Here's how the part is built. I have some questions about the finished solid (model axes, mm). A direction names the side the tool comes from. Round coordinates to 2 decimals unless told otherwise and drop trailing zeros. Write each loop counter-clockwise with the first axis right and the second up, starting at its lowest first coordinate (ties: lowest second). Pieces come first, ordered by that corner, then holes. Notation, with made-up numbers: (-36, 47) -> (-25, 47) arc R30 ccw to (-25, 84) -> close; hole circle Ø5 at (82, 58.5). An arc over 180 degrees is marked (long way). Put each result on its own line as item: value. Start each with the question number.
1) I want a section at C-C, the plane x = 59. List the corners of the cut face in (y, z) for me.
2) I want a section at A-A, the plane x = 38.5. List the corners of the cut face in (y, z) for me, then the cut area to 3 significant figures.
3) I want a section at B-B, the plane y = 0.35. Give the number of separate pieces and of enclosed holes in the cut face, then the cut area to 3 significant figures.
4) I want a section at D-D, the plane z = -5. List the corners of the cut face in (x, y) for me, then the cut area to 3 significant figures.
5) Which directions (+Z, -Z, +X, -X, +Y, -Y) give clear straight access to the entire face, cutting with the end or side of a thin tool? Please do faces 1 (the flat face through (5.1, 0.5, 159.9)), 2 (the flat face through (135.876, 0.493, 193.83)).
6) Will this pin go through, and if not, where does the flat tip stop? P1, Ø1.9, axis at x = 114.56, z = 121.63, coming from the -Y side (3 decimals).
7) We'd pull the mould along Z, two halves only. Please class faces 3 (the flat face through (4.93, 0.493, 244.636)), 4 (the flat face through (160, 1, -3)), 5 (the flat face through (5.2, 0.5, -159.8)): released by +Z, released by -Z, zero draft, split by the parting line, or undercut.
8) If I drill on line 1 along Z through (x, y) = (108, 0.6); line 2 along Z through (x, y) = (128, 0.6); line 3 along Z through (x, y) = (105, 0.5), over which ranges is the centre line in solid material (lowest first)? Write a range as [from, to].
from build123d import *

# Parameters (mm, degrees)
EXTRUDE_1_DEPTH     = 1
SKETCH_4_W          = 56.568542495
SKETCH_4_H          = 273.13708499
CUT_EXTRUDE_3_DEPTH = 354.138500868
CHAMFER_1_SIZE      = 10
SKETCH_5_R          = 1.6
CUT_EXTRUDE_4_DEPTH = 10
SKETCH_6_R          = 3
CUT_EXTRUDE_5_DEPTH = 10
SKETCH_7_R          = 1.6
CUT_EXTRUDE_6_DEPTH = 4


with BuildPart() as part:
    # 草图1 → 凸台-拉伸1 (new body)
    with BuildSketch(Plane(origin=(0, 0, 0), x_dir=(1, 0, 0), z_dir=(0, 1, 0))):
        with BuildLine():
            Line((0, 249.705627485), (0, 155))
            ThreePointArc((0, 155), (109.601551084, 109.601551084), (155, 0))
            ThreePointArc((155, 0), (109.601551084, -109.601551084), (0, -155))
            Line((0, -155), (0, -249.705627485))
            Line((0, -249.705627485), (80, -249.705627485))
            Line((80, -249.705627485), (249.705627485, -80))
            Line((249.705627485, -80), (249.705627485, 0))
            Line((249.705627485, 0), (249.705627485, 80))
            Line((249.705627485, 80), (80, 249.705627485))
            Line((80, 249.705627485), (0, 249.705627485))
        make_face()
    extrude(amount=EXTRUDE_1_DEPTH)

    # 草图4 → 切除-拉伸3 (cut, through all)
    with BuildSketch(Plane(origin=(0, 1, 0), x_dir=(1, 0, 0), z_dir=(0, 1, 0))):
        with Locations((221.421356237, 0)):
            Rectangle(SKETCH_4_W, SKETCH_4_H)
    extrude(amount=-CUT_EXTRUDE_3_DEPTH, mode=Mode.SUBTRACT)

    # 倒角1
    # the kernel refuses this chamfer: 10 mm, written as the material it takes off along each edge
    with BuildSketch(Plane(origin=(0, -26.617651024, -155), x_dir=(0.9994423420060535, 0, 0.0333916906648138), z_dir=(0, 1, 0))) as chamfer_1_piece_1:
        with BuildLine():
            Line((10.351424106, 0), (-CHAMFER_1_SIZE * 0.0333916906648, CHAMFER_1_SIZE * 0.999442342006))
            Line((-CHAMFER_1_SIZE * 0.0333916906648, CHAMFER_1_SIZE * 0.999442342006), (0, 0))
            ThreePointArc((0, 0), (5.321987279, 0.086367968), (10.351424106, 0))
        make_face()
    extrude(amount=54.235302047, mode=Mode.SUBTRACT)
    with BuildSketch(Plane(origin=(0, -25.71682988, -249.705627485), x_dir=(0, 0, 1), z_dir=(0, 1, 0))) as chamfer_1_piece_2:
        Polygon((CHAMFER_1_SIZE, 0), (0, CHAMFER_1_SIZE), (0, 0), align=None)
    extrude(amount=52.433659759, mode=Mode.SUBTRACT)
    with BuildSketch(Plane(origin=(80, -25.926703929, -249.705627485), x_dir=(-1, 0, 0), z_dir=(0, 1, 0)), Plane(origin=(193.13708499, 26.926703929, 136.568542495), x_dir=(-0.7071067811865447, 0, 0.7071067811865503), z_dir=(0, -1, 0))) as chamfer_1_piece_3:
        Polygon((CHAMFER_1_SIZE, 0), (-CHAMFER_1_SIZE * 0.707106781187, CHAMFER_1_SIZE * 0.707106781187), (0, 0), align=None)
    extrude(amount=52.853407858, mode=Mode.SUBTRACT)
    with BuildSketch(Plane(origin=(80, -25.926703929, 249.705627485), x_dir=(-1, 0, 0), z_dir=(0, 1, 0)), Plane(origin=(193.13708499, 26.926703929, -136.568542495), x_dir=(-0.7071067811865476, 0, -0.7071067811865476), z_dir=(0, -1, 0))) as chamfer_1_piece_4:
        Polygon((CHAMFER_1_SIZE, 0), (-CHAMFER_1_SIZE * 0.707106781187, -CHAMFER_1_SIZE * 0.707106781187), (0, 0), align=None)
    extrude(amount=52.853407858, mode=Mode.SUBTRACT)
    with BuildSketch(Plane(origin=(0, -25.71682988, 249.705627485), x_dir=(0, 0, -1), z_dir=(0, 1, 0))) as chamfer_1_piece_5:
        Polygon((CHAMFER_1_SIZE, 0), (0, -CHAMFER_1_SIZE), (0, 0), align=None)
    extrude(amount=52.433659759, mode=Mode.SUBTRACT)
    with BuildSketch(Plane(origin=(0, -26.617651024, 155), x_dir=(0, 0, 1), z_dir=(0, 1, 0))) as chamfer_1_piece_6:
        with BuildLine():
            Line((CHAMFER_1_SIZE, 0), (-0.345651552, 10.345651552))
            ThreePointArc((-0.345651552, 10.345651552), (-0.091390348, 5.321903403), (0, 0))
            Line((0, 0), (CHAMFER_1_SIZE, 0))
        make_face()
    extrude(amount=54.235302047, mode=Mode.SUBTRACT)

    # 草图5 → 切除-拉伸4 (cut)
    with BuildSketch(Plane(origin=(0, 1, 0), x_dir=(1, 0, 0), z_dir=(0, 1, 0))):
        with Locations(Location((98.03122292, -221.774909628, 0), (0, 0, 270))):
            Circle(SKETCH_5_R)
        with Locations(Location((108.637824638, -211.16830791, 0), (0, 0, 270))):
            Circle(SKETCH_5_R)
        with Locations(Location((154.599765415, -165.206367133, 0), (0, 0, 270))):
            Circle(SKETCH_5_R)
        with Locations(Location((165.206367133, -154.599765415, 0), (0, 0, 270))):
            Circle(SKETCH_5_R)
        with Locations(Location((165.206367133, 154.599765415, 0), (0, 0, 270))):
            Circle(SKETCH_5_R)
        with Locations(Location((154.599765415, 165.206367133, 0), (0, 0, 270))):
            Circle(SKETCH_5_R)
        with Locations(Location((108.637824638, 211.16830791, 0), (0, 0, 270))):
            Circle(SKETCH_5_R)
        with Locations(Location((98.03122292, 221.774909628, 0), (0, 0, 270))):
            Circle(SKETCH_5_R)
    extrude(amount=-CUT_EXTRUDE_4_DEPTH, mode=Mode.SUBTRACT)

    # 草图6 → 切除-拉伸5 (cut)
    with BuildSketch(Plane(origin=(0, 1, 0), x_dir=(1, 0, 0), z_dir=(0, 1, 0))):
        with Locations(Location((47.5, 242.75, 0), (0, 0, 270))):
            Circle(SKETCH_6_R)
        with Locations(Location((47.5, -242.75, 0), (0, 0, 270))):
            Circle(SKETCH_6_R)
    extrude(amount=-CUT_EXTRUDE_5_DEPTH, mode=Mode.SUBTRACT)

    # 草图7 → 切除-拉伸6 (cut)
    with BuildSketch(Plane(origin=(0, 1, 0), x_dir=(1, 0, 0), z_dir=(0, 1, 0))):
        with Locations(Location((114.557611845, 121.628679656, 0), (0, 0, 270))):
            Circle(SKETCH_7_R)
        with Locations(Location((128.699747468, 107.486544033, 0), (0, 0, 270))):
            Circle(SKETCH_7_R)
        with Locations(Location((128.699747468, -107.486544033, 0), (0, 0, 270))):
            Circle(SKETCH_7_R)
        with Locations(Location((114.557611845, -121.628679656, 0), (0, 0, 270))):
            Circle(SKETCH_7_R)
    extrude(amount=-CUT_EXTRUDE_6_DEPTH, mode=Mode.SUBTRACT)


solid = part.part
Findings:
1. outline: (0, -249.71) -> (1, -249.71) -> (1, -143.33) -> (0, -143.33) -> close; (0, 143.33) -> (1, 143.33) -> (1, 249.71) -> (0, 249.71) -> close
2. outline: (0, -249.71) -> (1, -249.71) -> (1, -150.14) -> (0, -150.14) -> close; (0, 150.14) -> (1, 150.14) -> (1, 249.71) -> (0, 249.71) -> close
2. area: 199 mm2
3. separate pieces: 1
3. enclosed holes: 14
3. area: 45,400 mm2
4. outline: (154.92, 0) -> (193.14, 0) -> (193.14, 1) -> (154.92, 1) -> close
4. area: 38.2 mm2
5. face 1: -X, +Y, -Y
5. face 2: +Z, +X, +Y, -Y
6. P1: passes through
7. face 3: released by +Z
7. face 4: zero draft
7. face 5: undercut
8. line 1: z = [-221.71, -212.64], [-209.7, -111.18], [111.18, 209.7], [212.64, 221.71]
8. line 2: z = [-201.71, -108.93], [-106.05, -87.41], [87.41, 106.05], [108.93, 201.71]
8. line 3: z = [-224.71, -114.02], [114.02, 224.71]
